Input: part model. Units: mm. Frame: model coordinates. A direction names the side the tool comes from. Round coordinates to 2 decimals unless told otherwise and drop trailing zeros. Loops run counter-clockwise (first coordinate to the right, second up) from the corner with the lowest first, then second, coordinate; pieces in that order, holes last. Notation, with made-up numbers: (-11, 54) - (-1, 54) arc R3 ccw to (-1, 59) - close; hole circle Ø4 at (34.25, 12). An arc over 180 degrees is marked (long way). Use CSV: the item, a comma, the result in double quotes. Start each with the question number.
1. Cut plane A-A (z = 2.75). Return loops of the section in (x, y), and give its area (3 significant figures).
2. Material intervals for probe 1 along Y at (x, z) = (0, 10.75); probe 2 along Y at (x, z) = (-40, 10); probe 3 along Y at (x, z) = (52, 13), sorted ascending. Write a range as from..to.
3. Pull-direction query (Y, two-part tool) for faces 3 (the flat face through (-1, 18, 15)), 4 (the flat face through (-1, -40, 7)), 5 (the cylindrical face through (-18, 14, 12)); classes: +Y half, -Y half, draft (parallel to the pull), parting line (faces both ways), or undercut.
4. Pin query (flat end, axial travel): P1, Ø3, axis at x = 52.5, y = -1, coming from the +Z side; P2, Ø15, axis at x = 1.5, y = 5.5, coming from the +Z side. Return the tip coordinate at first contact, or that it passes through.
5. Cut plane B-B (x = 52). Return loops of the section in (y, z).
6. Cut plane C-C (y = 25). Return loops of the section in (x, z), and give its area (3 significant figures).
7. Access query for faces 1 (the flat face through (20, 0, 12)), 2 (the cylindrical face through (37.05, -22.3, 7.6)). Directions: +Z, -Z, +X, -X, +Y, -Y. A direction counts if a zero-diameter tool reaches every point of the face in a straight line with its end or side. Return the directions, or none.
8. Cut plane D-D (x = -40). Return loops of the section in (y, z), and give its area (3 significant figures).
```python
from build123d import *

# Parameters (mm, degrees)
SKETCH_1_W          = 120
SKETCH_1_H          = 80
EXTRUDE_1_DEPTH     = 15
CUT_EXTRUDE_1_DEPTH = 6
SKETCH_3_R          = 4
CUT_EXTRUDE_2_DEPTH = 74.654599313
SKETCH_4_R          = 3
CUT_EXTRUDE_3_DEPTH = 10


with BuildPart() as part:
    # 草图1 → 凸台-拉伸1 (new body)
    with BuildSketch(Plane.XY):
        Rectangle(SKETCH_1_W, SKETCH_1_H)
    extrude(amount=EXTRUDE_1_DEPTH)

    # 草图2 → 切除-拉伸1 (cut)
    with BuildSketch(Plane.XY.offset(15)):
        with BuildLine():
            Line((-15, -15), (15, -15))
            ThreePointArc((15, -15), (18.535533906, -13.535533906), (20, -10))
            Line((20, -10), (20, 10))
            ThreePointArc((20, 10), (18.535533906, 13.535533906), (15, 15))
            Line((15, 15), (-15, 15))
            ThreePointArc((-15, 15), (-18.535533906, 13.535533906), (-20, 10))
            Line((-20, 10), (-20, -10))
            ThreePointArc((-20, -10), (-18.535533906, -13.535533906), (-15, -15))
        make_face()
    extrude(amount=-CUT_EXTRUDE_1_DEPTH, mode=Mode.SUBTRACT)

    # 草图3 → 切除-拉伸2 (cut, through all)
    with BuildSketch(Plane.XY.offset(15)):
        with Locations((0, 25)):
            Circle(SKETCH_3_R)
        with Locations((0, -25)):
            Circle(SKETCH_3_R)
        with Locations((40, 25)):
            Circle(SKETCH_3_R)
        with Locations((40, -25)):
            Circle(SKETCH_3_R)
        with Locations((-40, 25)):
            Circle(SKETCH_3_R)
        with Locations((-40, -25)):
            Circle(SKETCH_3_R)
    extrude(amount=-CUT_EXTRUDE_2_DEPTH, mode=Mode.SUBTRACT)

    # 草图4 → 切除-拉伸3 (cut)
    with BuildSketch(Plane.XY.offset(15)):
        with Locations((52, 0)):
            Circle(SKETCH_4_R)
        with Locations((-52, 0)):
            Circle(SKETCH_4_R)
    extrude(amount=-CUT_EXTRUDE_3_DEPTH, mode=Mode.SUBTRACT)


solid = part.part
```
Established:
1,outline,"(-60, -40) - (60, -40) - (60, 40) - (-60, 40) - close; hole circle Ø8 at (-40, -25); hole circle Ø8 at (-40, 25); hole circle Ø8 at (0, -25); hole circle Ø8 at (0, 25); hole circle Ø8 at (40, -25); hole circle Ø8 at (40, 25)"
1,area,"9,300 mm2"
2,probe 1,"y = -40..-29, -21..-15, 15..21, 29..40"
2,probe 2,"y = -40..-29, -21..21, 29..40"
2,probe 3,"y = -40..-3, 3..40"
3,face 3,"draft"
3,face 4,"-Y half"
3,face 5,"undercut"
4,P1,"stops at z = 5"
4,P2,"stops at z = 9"
5,outline,"(-40, 0) - (40, 0) - (40, 15) - (3, 15) - (3, 5) - (-3, 5) - (-3, 15) - (-40, 15) - close"
6,outline,"(-60, 0) - (-44, 0) - (-44, 15) - (-60, 15) - close; (-36, 0) - (-4, 0) - (-4, 15) - (-36, 15) - close; (4, 0) - (36, 0) - (36, 15) - (4, 15) - close; (44, 0) - (60, 0) - (60, 15) - (44, 15) - close"
6,area,"1,440 mm2"
7,face 1,"+Z"
7,face 2,"+Z, -Z"
8,outline,"(-40, 0) - (-29, 0) - (-29, 15) - (-40, 15) - close; (-21, 0) - (21, 0) - (21, 15) - (-21, 15) - close; (29, 0) - (40, 0) - (40, 15) - (29, 15) - close"
8,area,"960 mm2"
